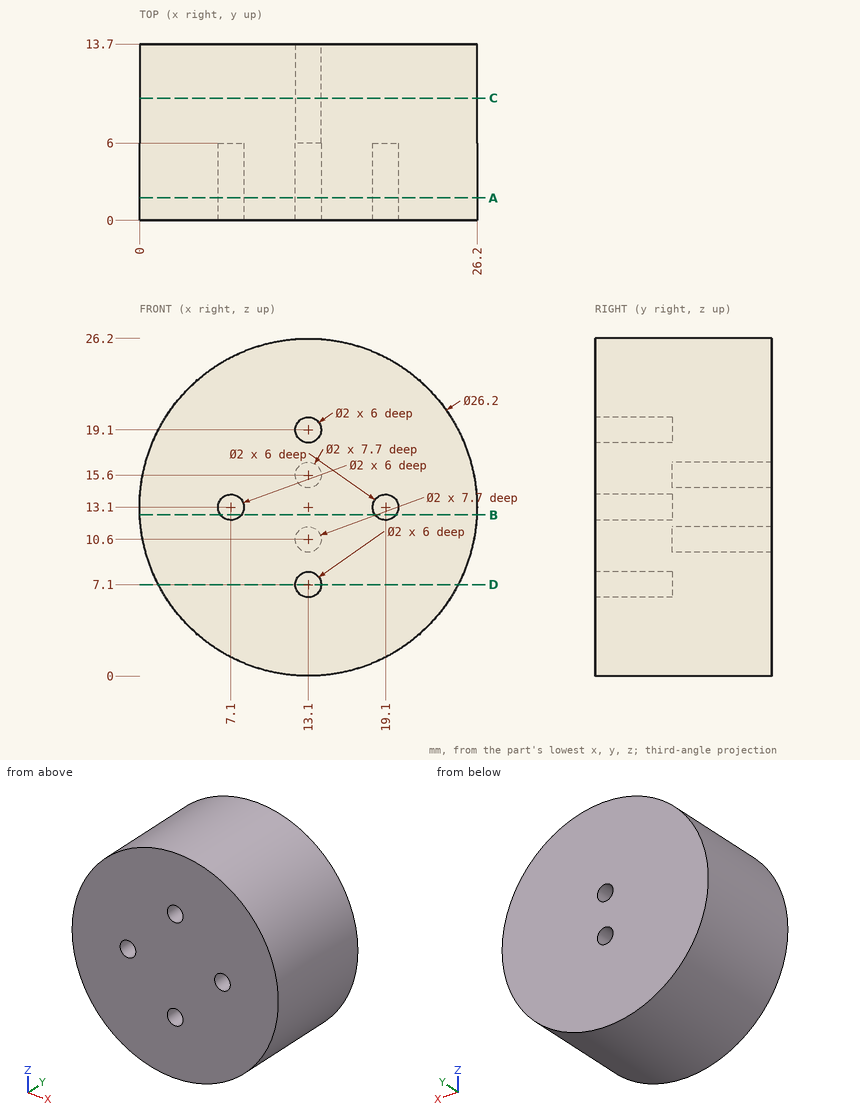
Input: dimensioned drawing with shaded views. Units: mm. Origin: part minimum x, y, z. Round coordinates to 2 decimals unless told otherwise and drop trailing zeros. Loops run counter-clockwise (first coordinate to the right, second up) from the corner with the lowest first, then second, coordinate; pieces in that order, holes last. Notation, with made-up numbers: (58.5, 82.5) -> (85.5, 82.5) arc R13 ccw to (85.5, 99.5) -> close; hole circle Ø5 at (5.5, 67.25). An arc over 180 degrees is marked (long way). Use one line per item in the form item = value. Start each with the question number.
1) Line query: L1, parallel to Z at x = 13.1, y = 2.45; L2, parallel to Z at x = 13.1, y = 9; L3, parallel to Z at x = 8, y = 2.5. Output: solid intervals per line, ascending.
2) Section B-B on z = 12.5. Output: boundary loops of the cut face in (x, y), then the cut area to 3 significant figures.
3) Section D-D on z = 7.1. Output: boundary loops of the cut face in (x, y).
4) First-contact query: P1, Ø8, axis at x = 17, y = 8.5, coming from the -Z side; P2, Ø3, axis at x = 4.5, y = 3.5, coming from the -Z side; P3, Ø5, axis at x = 9, y = 4, coming from the -Z side; P4, Ø1, axis at x = 13.5, z = 15.5, coming from the +Y side. Flat tips, straight axial feed; report the tip coordinate or a pass-through.
5) Section C-C on y = 9.5. Output: boundary loops of the cut face in (x, z).
6) Section A-A on y = 1.75. Output: boundary loops of the cut face in (x, z), then the cut area to 3 significant figures.
Response:
q1.L1 = 0 to 6.1, 8.1 to 18.1, 20.1 to 26.2
q1.L2 = 0 to 9.6, 11.6 to 14.6, 16.6 to 26.2
q1.L3 = 1.03 to 12.66, 13.54 to 25.17
q2.outline = (0.01, 0) -> (6.3, 0) -> (6.3, 6) -> (7.9, 6) -> (7.9, 0) -> (18.3, 0) -> (18.3, 6) -> (19.9, 6) -> (19.9, 0) -> (26.19, 0) -> (26.19, 13.7) -> (0.01, 13.7) -> close
q2.area = 339 mm^2
q3.outline = (1.45, 0) -> (12.1, 0) -> (12.1, 6) -> (14.1, 6) -> (14.1, 0) -> (24.75, 0) -> (24.75, 13.7) -> (1.45, 13.7) -> close
q4.P1 = 0
q4.P2 = 2.09
q4.P3 = 0.1
q4.P4 = 6
q5.outline = circle Ø26.2 at (13.1, 13.1); hole circle Ø2 at (13.1, 10.6); hole circle Ø2 at (13.1, 15.6)
q6.outline = circle Ø26.2 at (13.1, 13.1); hole circle Ø2 at (7.1, 13.1); hole circle Ø2 at (13.1, 7.1); hole circle Ø2 at (13.1, 19.1); hole circle Ø2 at (19.1, 13.1)
q6.area = 527 mm^2
